```python
from build123d import *

# Parameters (mm, degrees)
F1_DEPTH = 15
F2_W     = 5
F2_H     = 5
F3_DEPTH = 70
F5_DEPTH = 10


with BuildPart() as f1:
    # F0 (on Top) → F1 (new body)
    with BuildSketch(Plane.XY):
        with BuildLine():
            ThreePointArc((55, 65), (53.535534, 68.535534), (50, 70))
            Line((50, 70), (-50, 70))
            ThreePointArc((-50, 70), (-53.535534, 68.535534), (-55, 65))
            Line((-55, 65), (-55, -65))
            ThreePointArc((-55, -65), (-53.535534, -68.535534), (-50, -70))
            Line((-50, -70), (50, -70))
            ThreePointArc((50, -70), (53.535534, -68.535534), (55, -65))
            Line((55, -65), (55, 65))
        make_face()
    extrude(amount=F1_DEPTH)

    # F2 (on Front) → F3 (cut, symmetric)
    with BuildSketch(Plane.XZ):
        Polygon((-50, 5), (-45, 5), (-45, 10), (-55, 10), (-55, 5), align=None)
        with Locations((-52.5, 2.5)):
            Rectangle(F2_W, F2_H)
        with Locations((52.5, 2.5)):
            Rectangle(F2_W, F2_H)
        Polygon((50, 5), (55, 5), (55, 10), (45, 10), (45, 5), align=None)
    extrude(amount=F3_DEPTH, both=True, mode=Mode.SUBTRACT)

    # F4 (on face) → F5 (cut)
    with BuildSketch(Plane.XZ.offset(70)):
        Polygon((-50, 0), (50, 0), (50, 5), (45, 5), (45, 10), (-45, 10), (-45, 5), (-50, 5), align=None)
    extrude(amount=-F5_DEPTH, mode=Mode.SUBTRACT)


solid = f1.part
```
Input: part model. Units: mm. Frame: model coordinates. A direction names the side the tool comes from. Give positions to 0.01 mm unless a question says otherwise; leave off trailing zeros. Loops run counter-clockwise (first coordinate to the right, second up) from the corner with the lowest first, then second, coordinate; pieces in that order, holes last.
1) Section query B-B on x = 33.5. Return the cut outline in (y, z).
A:
outline: (-70, 10) - (-60, 10) - (-60, 0) - (70, 0) - (70, 15) - (-70, 15) - close
2) Line query: L1, parallel to Z at x = 47, y = 21; L2, parallel to Y at x = 36.5, z = 8; L3, parallel to X at y = -47.5, z = 4. Output: solid intervals per line, ascending.
A:
L1: z = 0 to 5, 10 to 15
L2: y = -60 to 70
L3: x = -50 to 50
3) Reachability of faces 1 (the flat face through (-45, 6, 7)), 2 (the flat face through (50, 4, 2)), 3 (the flat face through (-50, 6, 2)) from +Z, -Z, +X, -X, +Y, -Y: full face, straight path, thin tool, end or side. Return the list, or none.
A:
face 1: -X, +Y, -Y
face 2: -Z, +X, +Y, -Y
face 3: -Z, -X, +Y, -Y
4) Section query A-A on y = -35. Return the cut outline in (x, z), and give its area (3 significant figures).
A:
outline: (-55, 10) - (-45, 10) - (-45, 5) - (-50, 5) - (-50, 0) - (50, 0) - (50, 5) - (45, 5) - (45, 10) - (55, 10) - (55, 15) - (-55, 15) - close
area: 1,500 mm2
5) Mould query, pull axis Z, two halves, no side actions, for faces 4 (the flat face through (-1, 6, 0)), 5 (the flat face through (45, 4, 8)), 6 (the cylindrical face through (54, 68, 12)), 7 (the flat face through (49, -10, 10)). Classes: released by +Z, released by -Z, zero draft, split by the parting line, or undercut.
A:
face 4: released by -Z
face 5: undercut
face 6: zero draft
face 7: undercut
6) Contact query for flat-ended pins moving along their axis: pin 1 (2.5 mm diameter, centred on y = -0.5, z = 1.5, fed in from +X); pin 2 (8 mm diameter, centred on x = 20.5, z = 3, fed in from -Y); pin 3 (5 mm diameter, centred on y = -6.5, z = 4.5, fed in from -X). Output: stop coordinate, or through.
A:
pin 1: stops at x = 50
pin 2: stops at y = -60
pin 3: stops at x = -50
